from build123d import *

# Parameters (mm, degrees)
BOSS_EXTRUDE1_DEPTH = 30
CUT_EXTRUDE1_DEPTH  = 16
CUT_EXTRUDE3_DEPTH  = 8
CUT_EXTRUDE4_DEPTH  = 10


with BuildPart() as part:
    # Sketch1 → Boss-Extrude1 (new, symmetric)
    with BuildSketch(Plane.XY):
        with BuildLine():
            Line((0, 0), (0, 20))
            Line((0, 20), (0, 50))
            Line((0, 50), (48, 50))
            Line((48, 50), (60, 50))
            Line((60, 50), (60, 30))
            Line((60, 30), (100, 30))
            Line((100, 30), (100, 0))
            Line((100, 0), (66, 0))
            ThreePointArc((66, 0), (48, 18), (30, 0))
            Line((30, 0), (0, 0))
        make_face()
    extrude(amount=BOSS_EXTRUDE1_DEPTH, both=True)

    # Sketch2 → Cut-Extrude1 (cut)
    with BuildSketch(Plane.XY.offset(30)):
        Polygon((0, 20), (48, 50), (0, 50), align=None)
    cut_extrude1 = extrude(amount=-CUT_EXTRUDE1_DEPTH, mode=Mode.SUBTRACT)

    # Mirror1: Cut-Extrude1 across plane
    add(cut_extrude1.mirror(Plane.XY), mode=Mode.SUBTRACT)

    # Sketch4 → Cut-Extrude3 (cut, symmetric)
    with BuildSketch(Plane.XY):
        with BuildLine():
            Line((60, 50), (31.510004003, 50))
            ThreePointArc((31.510004003, 50), (42.210944462, 34.902981487), (60, 40))
            Line((60, 40), (60, 50))
        make_face()
    extrude(amount=CUT_EXTRUDE3_DEPTH, both=True, mode=Mode.SUBTRACT)

    # Sketch5 → Cut-Extrude4 (cut, symmetric)
    with BuildSketch(Plane.XY):
        Polygon((100, 0), (100, 30), (70, 30), align=None)
    extrude(amount=CUT_EXTRUDE4_DEPTH, both=True, mode=Mode.SUBTRACT)


solid = part.part
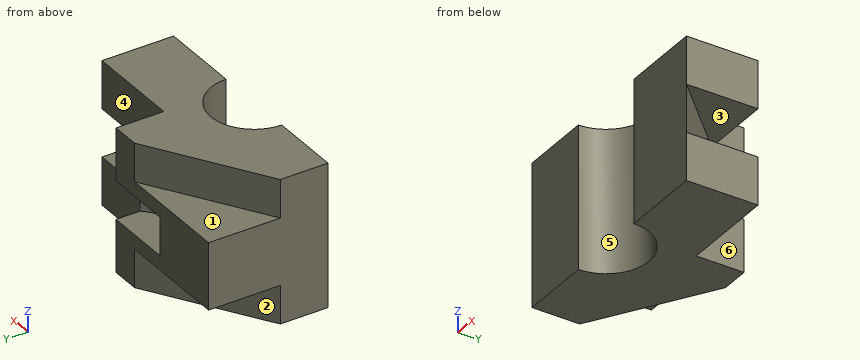
Can you work these out from the model? Positions are in its coordinate system, mm. Face numbers are marked on the shaded views. A direction names the side the tool comes from. Round coordinates to 2 decimals unless told otherwise and drop trailing zeros. Write each loop counter-clockwise with the first axis right and the second up, starting at its lowest first coordinate (ties: lowest second). Pieces come first, ordered by that corner, then holes. Notation, with made-up numbers: M 75,15 L 112,15 A22 cw 112,23 Z; hole C 55,6 d10. An arc over 180 degrees is marked long. Use CSV: the item, a comma, the result in double quotes.
(1) On a 3-axis mill with a long thin cutter (end or side, diameter ignored), from which of +Z, -Z, +X, -X, +Y, -Y can I reach the whole of each face in a straight line? I mean the marked faces 1, 2 and 3. Say none if no direction works.
Check values:
face 1,"+Z, -X, +Y"
face 2,"-Z, -X, +Y"
face 3,"+X, +Y"
(2) Imagine slicing it at A-A (x = 85.5). Write out the boundary of the cut face in (y, z).
Check values:
outline,"M 0,-30 L 30,-30 L 30,-10 L 14.5,-10 L 14.5,10 L 30,10 L 30,30 L 0,30 Z"
(3) Imagine slicing it at D-D (y = 43). Write out the boundary of the cut face in (x, z), plus the area to 3 significant figures.
Check values:
outline,"M 0,-14 L 36.8,-14 L 36.8,-30 L 60,-30 L 60,-8 L 33.12,-8 L 33.12,8 L 60,8 L 60,30 L 36.8,30 L 36.8,14 L 0,14 Z"
area,"1,990 mm^2"
(4) We'd pull the mould along X, two halves only. Please class the marked faces 4, 5 and 6: +X half, -X half, draft (parallel to the pull), parting line (faces both ways), or undercut.
Check values:
face 4,"draft"
face 5,"undercut"
face 6,"+X half"
(5) Imagine slicing it at C-C (z = 21). Write out the boundary of the cut face in (x, y), plus the area to 3 significant figures.
Check values:
outline,"M 0,0 L 30,0 A18 cw 66,0 L 100,0 L 100,30 L 60,30 L 60,50 L 48,50 L 0,20 Z"
area,"2,970 mm^2"
(6) I need wall thicknesses on line 1 along Z through (x, y) = (45, 39); line 2 along Z through (x, y) = (81, 21); line 3 along Z through (x, y) = (10, 47.5). Which ranges of each line are inside material? Lowest first, please.
Check values:
line 1,"-30 to -8, 8 to 30"
line 2,"-30 to -10, 10 to 30"
line 3,"-14 to 14"
(7) I'm going to push flat-ended pins straight in: pin 1 (10 mm diameter, centred on y = 39.5, z = -14.5, fed in from +X); pin 2 (3 mm diameter, centred on y = 8, z = -4, fed in from +X); pin 3 (20 mm diameter, centred on x = 72, z = 12, fed in from +Y). Where does each tip first touch, or does it pass through?
Check values:
pin 1,"x = 60"
pin 2,"x = 93.5"
pin 3,"y = 30"
(8) Imagine slicing it at B-B (y = 37.5). Write out the boundary of the cut face in (x, z).
Check values:
outline,"M 0,-14 L 28,-14 L 28,-30 L 60,-30 L 60,30 L 28,30 L 28,14 L 0,14 Z; hole M 37.52,-8 L 57.5,-8 L 57.5,8 L 37.52,8 Z"
